Autodesk Inventor part; units mm, degrees
ref_plane "작업 평면1" through (0, 0, 12.5) normal (0, 0, 1) x (1, 0, 0)
ref_plane "작업 평면2" through (0, 20, 0) normal (0, -1, 0) x (1, 0, 0)
ref_plane "YZ Plane" through (0, 0, 0) normal (1, 0, 0) x (0, 1, 0)
sketch "스케치1" plane through (0, 0, 0) normal (0, 0, 1) x (1, 0, 0)
  line L0 (0, 0) -> (60, 0)
  line L1 (60, 0) -> (60, 40)
  line L2 (60, 40) -> (0, 40)
  line L3 (0, 40) -> (0, 0)
  dimension "d0" = 40
  dimension "d1" = 60
extrude "돌출1" add sketch "스케치1" along normal blind 25
sketch "스케치2" plane through (0, 0, 25) normal (0, 0, 1) x (1, 0, 0)
  line L0 (60, 0) -> (60, 40)
  line L1 (60, 40) -> (0, 40)
  line L2 (0, 40) -> (0, 0)
  line L3 (0, 0) -> (60, 0)
  circle A0 centre (20, 20) radius 15
  point P0 (0, 20)
  dimension "d4" = 30
  dimension "d5" = 20
extrude "돌출2" cut sketch "스케치2" against normal through all contours A0
ref_plane "작업 평면1" through (0, 0, 12.5) normal (0, 0, 1) x (1, 0, 0)
ref_plane "작업 평면2" through (0, 20, 0) normal (0, -1, 0) x (1, 0, 0)
sketch "스케치3" plane through (60, 0, 0) normal (1, 0, 0) x (0, 0, -1)
  line L0 (0, 0) -> (0, 40)
  line L1 (0, 40) -> (-25, 40)
  line L2 (-25, 0) -> (-25, 40)
  line L3 (0, 0) -> (-25, 0)
  line L4 (-27.5, 0) -> (2.5, 0)
  line L5 (2.5, 0) -> (2.5, 40)
  line L6 (2.5, 40) -> (-27.5, 40)
  line L7 (-27.5, 40) -> (-27.5, 0)
  line L8 (-27.5, -8) -> (2.5, -8)
  line L9 (2.5, -8) -> (2.5, 48)
  line L10 (2.5, 48) -> (-27.5, 48)
  line L11 (-27.5, 48) -> (-27.5, -8)
  circle A0 centre (-16.5, -5) radius 1.5
  circle A1 centre (-2.5, -5) radius 1.5
  circle A2 centre (-16.5, 45) radius 1.5
  circle A3 centre (-2.5, 45) radius 1.5
  point P0 (0, 0)
  point P1 (-12.5, 0)
  point P2 (-12.5, 0)
  point P3 (-27.5, 20)
  point P4 (-25, 20)
  point P5 (-27.5, 0)
  point P6 (2.5, 0)
  dimension "d8" = 40
  dimension "d9" = 30
  dimension "d10" = 8
  dimension "d11" = 8
  dimension "d12" = 30
  dimension "d13" = 3
  dimension "d14" = 3
  dimension "d15" = 3
  dimension "d16" = 3
  dimension "d17" = 5
  dimension "d18" = 5
  dimension "d19" = 14
  dimension "d20" = 5
extrude "돌출3" add sketch "스케치3" along normal blind 5
properties part number "다리-0"
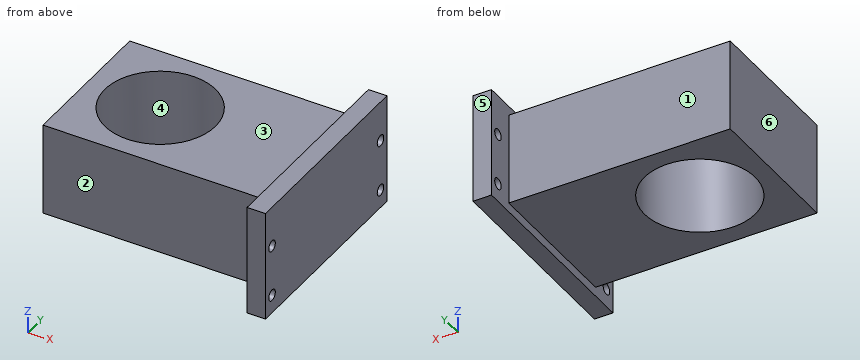
CAD build for the part. Positions are in the model's coordinates, mm. Face numbers are marked on the shaded views. A direction names the side the tool comes from. Round coordinates to 2 decimals unless told otherwise and drop trailing zeros. Write each loop counter-clockwise with the first axis right and the second up, starting at its lowest first coordinate (ties: lowest second). Pieces come first, ordered by that corner, then holes. Notation, with made-up numbers: (-23.75, -36.75) -> (18.25, -36.75) arc R20 ccw to (18.25, -21.75) -> close; hole circle Ø5 at (9, 17). An arc over 180 degrees is marked (long way). Answer as a JSON object with one key per item and string values.
(1) Pin check, flat tips, straight feed: P1, Ø2, axis at x = 41, y = 10.5, coming from the +Z side; P2, Ø20, axis at x = 43.5, y = 13, coming from the -Z side; P3, Ø4, axis at y = -5, z = 2.5, coming from the -X side; P4, Ø2, axis at y = 5, z = 16, coming from the -X side. Stop position of each tip, or through.
Reported:
{"P1": "stops at z = 25", "P2": "stops at z = 0", "P3": "stops at x = 60", "P4": "stops at x = 0"}
(2) Band-saw the part on A-A, the plane x = 29. List the corners of the cut face in (y, z), then the cut area to 3 significant figures.
Reported:
{"outline": "(0, 0) -> (8, 0) -> (8, 25) -> (0, 25) -> close; (32, 0) -> (40, 0) -> (40, 25) -> (32, 25) -> close", "area": "400 mm^2"}
(3) Probe probe 1 along Y at (x, z) = (62.9, 2.5); probe 2 along Y at (x, z) = (20, 16); probe 3 along Z at (x, y) = (22.5, 38). List the from-to ranges inside material, lowest first. Write a range as [from, to].
Reported:
{"probe 1": "y = [-8, -6.5], [-3.5, 43.5], [46.5, 48]", "probe 2": "y = [0, 5], [35, 40]", "probe 3": "z = [0, 25]"}
(4) Which spindle directions (+Z, -Z, +X, -X, +Y, -Y) get a long thin tool onto all of the face, cutting with end or side? Do the marked faces 1, 2 and 3. Say none if no direction does.
Reported:
{"face 1": "+Z, -Z, -X, +Y", "face 2": "+Z, -Z, -X, -Y", "face 3": "+Z, -X, +Y, -Y"}
(5) Band-saw the part on B-B, the plane z = 16.5. List the corners of the cut face in (x, y).
Reported:
{"outline": "(0, 0) -> (60, 0) -> (60, -3.5) -> (65, -3.5) -> (65, 43.5) -> (60, 43.5) -> (60, 40) -> (0, 40) -> close; (60, -8) -> (65, -8) -> (65, -6.5) -> (60, -6.5) -> close; (60, 46.5) -> (65, 46.5) -> (65, 48) -> (60, 48) -> close; hole circle Ø30 at (20, 20)"}
(6) Two-plate mould, pull along X, no slides. Class the marked faces 4, 5 and 6: +X half, -X half, draft (parallel to the pull), parting line (faces both ways), or undercut.
Reported:
{"face 4": "undercut", "face 5": "draft", "face 6": "-X half"}
(7) Band-saw the part on D-D, the plane y = 20. List the corners of the cut face in (x, z).
Reported:
{"outline": "(0, 0) -> (5, 0) -> (5, 25) -> (0, 25) -> close; (35, 0) -> (60, 0) -> (60, -2.5) -> (65, -2.5) -> (65, 27.5) -> (60, 27.5) -> (60, 25) -> (35, 25) -> close"}
(8) Band-saw the part on C-C, the plane y = -5. List the corners of the cut face in (x, z), then the cut area to 3 significant figures.
Reported:
{"outline": "(60, -2.5) -> (65, -2.5) -> (65, 1) -> (60, 1) -> close; (60, 4) -> (65, 4) -> (65, 15) -> (60, 15) -> close; (60, 18) -> (65, 18) -> (65, 27.5) -> (60, 27.5) -> close", "area": "120 mm^2"}
